Geometry: final body of the model. Coordinates: model frame, mm. Round coordinates to 2 decimals unless told otherwise and drop trailing zeros. Loops run counter-clockwise (first coordinate to the right, second up) from the corner with the lowest first, then second, coordinate; pieces in that order, holes last. Notation, with made-up numbers: (15.25, 18.25) -> (26.25, 18.25) arc R18 ccw to (26.25, 36.25) -> close; hole circle Ø10 at (-16.5, 70). An arc over 180 degrees is marked (long way). Answer in a Markdown table with one row per item.
```python
from build123d import *

# Parameters (mm, degrees)
SKETCH1_R          = 6
BASE_FLANGE1_DEPTH = 3


# Sheet-metal steps are written as plain solids
with BuildPart() as part:
    # Sketch1 → Base-Flange1 (new body)
    with BuildSketch(Plane.XY):
        with BuildLine():
            Line((-12.5, 29), (-12.5, -29))
            ThreePointArc((-12.5, -29), (0, -18.544994432), (12.5, -29))
            Line((12.5, -29), (12.5, 29))
            ThreePointArc((12.5, 29), (0, 35.708438024), (-12.5, 29))
        make_face()
        with Locations((0, 20.708438024)):
            Circle(SKETCH1_R, mode=Mode.SUBTRACT)
    extrude(amount=-BASE_FLANGE1_DEPTH)


solid = part.part
```
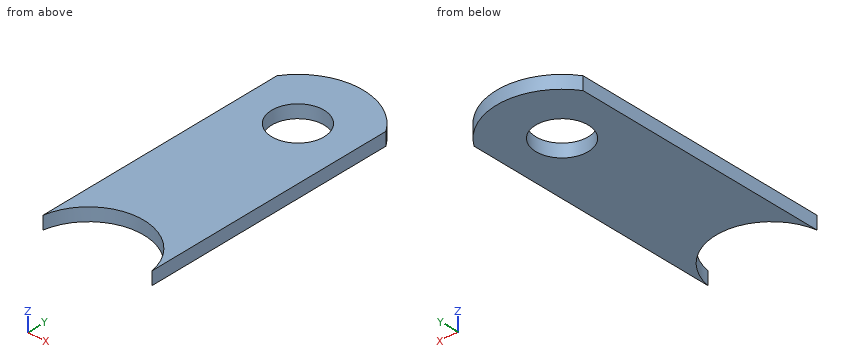
Item 1: Cut plane C-C (y = 32.5). Output: boundary loops of the cut face in (x, z).
Answer:
| item | result |
|---|---|
| outline | (-9.27, -3) -> (9.27, -3) -> (9.27, 0) -> (-9.27, 0) -> close |
Item 2: Line query: probe 1 along X at (y, z) = (22.5, -0.85); probe 2 along Y at (x, z) = (3.75, -2.55); probe 3 along Y at (x, z) = (3.25, -0.2). Output: solid intervals per line, ascending. Write a range as [from, to].
Answer:
| item | result |
|---|---|
| probe 1 | x = [-12.5, -5.73], [5.73, 12.5] |
| probe 2 | y = [-19.11, 16.02], [25.39, 35.23] |
| probe 3 | y = [-18.97, 15.66], [25.75, 35.35] |
Item 3: Cut plane B-B (z = -1.1). Output: boundary loops of the cut face in (x, y) (3 decimals), then the cut area to 3 significant figures.
Answer:
| item | result |
|---|---|
| outline | (-12.5, -29) arc R12.7 cw to (12.5, -29) -> (12.5, 29) arc R15 ccw to (-12.5, 29) -> close; hole circle Ø12 at (0, 20.708) |
| area | 1,260 mm² |
Item 4: Pin query (flat end, axial travel): pin 1 Ø1 at (x, z) = (5.5, -2.5) entering from +Y; pin 2 Ø1.5 at (x, z) = (1.5, -2.5) entering from +Y; pin 3 Ø10 at (x, y) = (1.5, 25) entering from +Z; pin 4 Ø11 at (x, y) = (0, 20.71) entering from -Z. Return the tip coordinate at first contact, or that it passes through.
Answer:
| item | result |
|---|---|
| pin 1 | stops at y = 34.85 |
| pin 2 | stops at y = 35.69 |
| pin 3 | stops at z = 0 |
| pin 4 | passes through |
Item 5: Cut plane A-A (x = 0). Output: boundary loops of the cut face in (y, z) (3 decimals), then the cut area to 3 significant figures.
Answer:
| item | result |
|---|---|
| outline | (-18.545, -3) -> (14.708, -3) -> (14.708, 0) -> (-18.545, 0) -> close; (26.708, -3) -> (35.708, -3) -> (35.708, 0) -> (26.708, 0) -> close |
| area | 127 mm² |
Item 6: Cut plane D-D (x = -8.25). Output: boundary loops of the cut face in (y, z), then the cut area to 3 significant figures.
Answer:
| item | result |
|---|---|
| outline | (-21.59, -3) -> (33.24, -3) -> (33.24, 0) -> (-21.59, 0) -> close |
| area | 164 mm² |
